Design review of the part built by this model. Coordinates are the model's own, in mm. A direction names the side the tool comes from. Round coordinates to 2 decimals unless told otherwise and drop trailing zeros. Loops run counter-clockwise (first coordinate to the right, second up) from the corner with the lowest first, then second, coordinate; pieces in that order, holes last. Notation, with made-up numbers: M 7.25,20.5 L 33.25,20.5 A24 ccw 33.25,38.5 Z; hole C -35,54.5 d3. An arc over 180 degrees is marked long. Answer as CSV lines item,"result". Start each with the question number.
from build123d import *

# Parameters (mm, degrees)
SKETCH1_W           = 100.5
SKETCH1_H           = 60.9
BOSS_EXTRUDE1_DEPTH = 1.8
SKETCH2_R           = 1.75
CUT_EXTRUDE1_DEPTH  = 1.8
SKETCH3_W           = 12
SKETCH3_H           = 12
BOSS_EXTRUDE2_DEPTH = 1.61
SKETCH4_W           = 7.5
SKETCH4_H           = 5.5
BOSS_EXTRUDE3_DEPTH = 2.5


with BuildPart() as part:
    # Sketch1 → Boss-Extrude1 (new body)
    with BuildSketch(Plane.XY):
        with Locations((0, 30.45)):
            Rectangle(SKETCH1_W, SKETCH1_H)
    extrude(amount=BOSS_EXTRUDE1_DEPTH)

    # Sketch2 → Cut-Extrude1 (cut)
    with BuildSketch(Plane.XY.offset(1.8)):
        with Locations((-46.25, 3.8)):
            Circle(SKETCH2_R)
        with Locations((-46.25, 57.1)):
            Circle(SKETCH2_R)
    cut_extrude1 = extrude(amount=-CUT_EXTRUDE1_DEPTH, mode=Mode.SUBTRACT)

    # Mirror1: Cut-Extrude1 across plane
    add(cut_extrude1.mirror(Plane(origin=(0, 0, 0), x_dir=(0, 0, 1), z_dir=(1, 0, 0))), mode=Mode.SUBTRACT)

    # Sketch3 → Boss-Extrude2 (add)
    with BuildSketch(Plane.XY.offset(1.8)):
        with Locations((36.25, 6)):
            Rectangle(SKETCH3_W, SKETCH3_H)
    extrude(amount=BOSS_EXTRUDE2_DEPTH)

    # Sketch4 → Boss-Extrude3 (add)
    with BuildSketch(Plane.XY.offset(1.8)):
        with Locations((-37.5, 1.25)):
            Rectangle(SKETCH4_W, SKETCH4_H)
    extrude(amount=BOSS_EXTRUDE3_DEPTH)


solid = part.part
Item 1: Consider section B-B, the plane x = -46.25. Write out the cut boundary in (y, z).
Item 2: Insertion check: pin 1 Ø1 at (x, z) = (18, 2) entering from -Y; pin 2 Ø0.8 at (x, z) = (-36, 3) entering from +Y; pin 3 Ø1.2 at (y, z) = (2, 3) entering from -X. Each pin has a flat end and moves straight along its axis. Give the tip position at first contact, or say it passes through.
Item 3: Consider section A-A, the plane y = 57.1. Write out the cut boundary in (x, z).
Item 4: Consider section C-C, the plane y = 14. Write out the cut boundary in (x, z), then the cut area to 3 significant figures.
Item 5: Consider section D-D, the plane x = 25.5. Write out the cut boundary in (y, z), then the cut area to 3 significant figures.
Item 6: Tool access review of faces 1 (the face through (-41.25, 1, 3)), 2 (the face through (-38, 4, 3)), 3 (the face through (-33.75, 1, 3)), 4 (the face through (36, 6, 3.41)): name each direction out of +Z, -Z, +X, -X, +Y, -Y from which nothing blocks a thin tool from reaching the whole face with its end or side.
Item 7: The part is to be moulded in two halves that separate along Y. For faces 5 (the face through (44.633, 3.13, 0.913)), 6 (the face through (-1, 60.9, 1)), 7 (the face through (50.25, 30, 1)), say which applies: +Y half, -Y half, draft (parallel to the pull), parting line (faces both ways), or undercut.
Item 8: To check wall thickness, follow line 1 (Y direction, x = 46.25, z = 0.8); line 2 (X direction, y = 3.5, z = 1.25); line 3 (Y direction, x = -10.5, z = 1.1). State the ranges of each line that lie inside material, in increasing order.
Found:
1,outline,"M 0,0 L 2.05,0 L 2.05,1.8 L 0,1.8 Z; M 5.55,0 L 55.35,0 L 55.35,1.8 L 5.55,1.8 Z; M 58.85,0 L 60.9,0 L 60.9,1.8 L 58.85,1.8 Z"
2,pin 1,"stops at y = 0"
2,pin 2,"stops at y = 4"
2,pin 3,"stops at x = -41.25"
3,outline,"M -50.25,0 L -48,0 L -48,1.8 L -50.25,1.8 Z; M -44.5,0 L 44.5,0 L 44.5,1.8 L -44.5,1.8 Z; M 48,0 L 50.25,0 L 50.25,1.8 L 48,1.8 Z"
4,outline,"M -50.25,0 L 50.25,0 L 50.25,1.8 L -50.25,1.8 Z"
4,area,"181 mm^2"
5,outline,"M 0,0 L 60.9,0 L 60.9,1.8 L 0,1.8 Z"
5,area,"110 mm^2"
6,face 1,"+Z, -X, +Y, -Y"
6,face 2,"+Z, -X, +Y"
6,face 3,"+Z, +Y, -Y"
6,face 4,"+Z, +X, +Y, -Y"
7,face 5,"undercut"
7,face 6,"+Y half"
7,face 7,"draft"
8,line 1,"y = 0 to 2.05, 5.55 to 55.35, 58.85 to 60.9"
8,line 2,"x = -50.25 to -47.97, -44.53 to 44.53, 47.97 to 50.25"
8,line 3,"y = 0 to 60.9"
